from build123d import *

# Parameters (mm, degrees)
BOSS_EXTRUDE3_DEPTH = 13
FILLET1_R           = 1
FILLET2_R           = 5
SKETCH2_R           = 2.4
CUT_EXTRUDE1_DEPTH  = 7.5
FILLET3_R           = 2.5


with BuildPart() as part:
    # Sketch1 → Boss-Extrude3 (new body)
    with BuildSketch(Plane.XY):
        Polygon((-12.5, 10.5), (-4.45, 10.5), (4.45, 10.5), (12.5, 10.5), (12.5, 24.5), (-12.5, 33.5), align=None)
        Polygon((-4.45, 7.3), (-10.25, 7.3), (-4, 0), (4, 0), (10.25, 7.3), (4.45, 7.3), (4.45, 10.5), (-4.45, 10.5), align=None)
    extrude(amount=BOSS_EXTRUDE3_DEPTH)

    # Fillet1
    fillet1_edges = [part.edges().sort_by_distance(p)[0] for p in [
        (10.25, 7.3, 6.5),
        (-10.25, 7.3, 6.5),
    ]]
    fillet(fillet1_edges, radius=FILLET1_R)

    # Fillet2
    fillet2_edges = [part.edges().sort_by_distance(p)[0] for p in [
        (4, 0, 6.5),
        (-4, 0, 6.5),
    ]]
    fillet(fillet2_edges, radius=FILLET2_R)

    # Sketch2 → Cut-Extrude1 (cut)
    with BuildSketch(Plane(origin=(9.242209632, 25.672804533, 0), x_dir=(0.9408874118687268, -0.33871946827274163, 0), z_dir=(0.33871946827274163, 0.9408874118687268, 0))):
        with Locations(Location((-17.537534324, -6.5, 0), (0, 0, 180))):
            Circle(SKETCH2_R)
        with Locations(Location((-2.537534324, -6.5, 0), (0, 0, 180))):
            Circle(SKETCH2_R)
    extrude(amount=-CUT_EXTRUDE1_DEPTH, mode=Mode.SUBTRACT)

    # Fillet3
    fillet3_edges = [part.edges().sort_by_distance(p)[0] for p in [
        (-12.5, 22, 13),
        (-12.5, 22, 0),
        (12.5, 17.5, 0),
        (12.5, 17.5, 13),
    ]]
    fillet(fillet3_edges, radius=FILLET3_R)


solid = part.part
Can you work these out from the model? Positions are in its coordinate system, mm. A direction names the side the tool comes from. Coordinates: 2 decimals unless noted, no trailing zeros. Write each loop counter-clockwise with the first axis right and the second up, starting at its lowest first coordinate (ties: lowest second). Pieces come first, ordered by that corner, then holes. Notation, with made-up numbers: (56.25, -14) - (103.25, -14) arc R29 ccw to (103.25, 24) - close; hole circle Ø11 at (-16.5, 87.25). An arc over 180 degrees is marked (long way). Return JSON: item names as keys, results as strings. Group by question number.
Item 1: I'm going to push flat-ended pins straight in: pin 1 Ø3.5 at (y, z) = (9.5, 7) entering from -X; pin 2 Ø6 at (x, z) = (9, 9.5) entering from +Y; pin 3 Ø4 at (x, z) = (-7, 8) entering from +Y; pin 4 Ø4 at (x, z) = (7.5, 3) entering from -Y. Where does each tip first touch, or does it pass through?
Item 2: Which directions (+Z, -Z, +X, -X, +Y, -Y) give clear straight access to the entire face, cutting with the end or side of a thin tool? Please do faces 1 (the face through (-6, 7.3, 6)), 2 (the face through (6, 7.3, 6)), 3 (the face through (-7.19, 3.726, 6.409)), 4 (the face through (-9.767, 24.545, 6.534)), 5 (the face through (7.14, 3.67, 6.41)).
Item 3: If we section it at C-C (z = 1): Write out the boundary of the cut face in (x, y), then the cut area to 3 significant figures.
Item 4: We'd pull the mould along X, two halves only. Please class faces 6 (the face through (4.45, 9, 6)), 7 (the face through (-6.255, 27.322, 6.606)), 8 (the face through (-12, 22, 12)): pulls with the +X half, pulls with the -X half, needs draft (parallel to the pull), parting line crosses it, or undercut.
Item 5: If we section it at B-B (z = 3): Write out the boundary of the cut face in (x, y).
Item 6: If we section it at A-A (y = 16): Write out the boundary of the cut face in (x, z), then the cut area to 3 significant figures.
Item 7: If we section it at D-D (z = 8.5): Write out the boundary of the cut face in (x, y), then the cut area to 3 significant figures.
Item 8: Please list where these lines run through material, in increasing order: probe 1 along Y at (x, z) = (8.5, 10); probe 2 along Y at (x, z) = (7, 2.5); probe 3 along Z at (x, y) = (-7, 27.5).
Return value:
{
 "1": {"pin 1": "stops at x = -12.5", "pin 2": "stops at y = 26.84", "pin 3": "stops at y = 32.24", "pin 4": "stops at y = 1.75"},
 "2": {"face 1": "+Z, -Z, -X", "face 2": "+Z, -Z, +X", "face 3": "+Z, -Z, -X, -Y", "face 4": "none", "face 5": "+Z, -Z, +X, -Y"},
 "3": {"outline": "(-12, 10.5) - (-4.45, 10.5) - (-4.45, 7.3) - (-8.08, 7.3) arc R1 ccw to (-8.84, 5.65) - (-5.5, 1.75) arc R5 ccw to (-1.7, 0) - (1.7, 0) arc R5 ccw to (5.5, 1.75) - (8.84, 5.65) arc R1 ccw to (8.08, 7.3) - (4.45, 7.3) - (4.45, 10.5) - (12, 10.5) - (12, 24.68) - (-12, 33.32) - close", "area": "573 mm^2"},
 "4": {"face 6": "pulls with the +X half", "face 7": "undercut", "face 8": "pulls with the -X half"},
 "5": {"outline": "(-12.5, 10.5) - (-4.45, 10.5) - (-4.45, 7.3) - (-8.08, 7.3) arc R1 ccw to (-8.84, 5.65) - (-5.5, 1.75) arc R5 ccw to (-1.7, 0) - (1.7, 0) arc R5 ccw to (5.5, 1.75) - (8.84, 5.65) arc R1 ccw to (8.08, 7.3) - (4.45, 7.3) - (4.45, 10.5) - (12.5, 10.5) - (12.5, 24.5) - (-12.5, 33.5) - close"},
 "6": {"outline": "(-12.5, 2.5) arc R2.5 ccw to (-10, 0) - (10, 0) arc R2.5 ccw to (12.5, 2.5) - (12.5, 10.5) arc R2.5 ccw to (10, 13) - (-10, 13) arc R2.5 ccw to (-12.5, 10.5) - close", "area": "320 mm^2"},
 "7": {"outline": "(-12.5, 10.5) - (-4.45, 10.5) - (-4.45, 7.3) - (-8.08, 7.3) arc R1 ccw to (-8.84, 5.65) - (-5.5, 1.75) arc R5 ccw to (-1.7, 0) - (1.7, 0) arc R5 ccw to (5.5, 1.75) - (8.84, 5.65) arc R1 ccw to (8.08, 7.3) - (4.45, 7.3) - (4.45, 10.5) - (12.5, 10.5) - (12.5, 24.5) - (8.1, 26.08) - (5.56, 19.03) - (3.07, 19.93) - (5.61, 26.98) - (-6.01, 31.16) - (-8.55, 24.11) - (-11.05, 25.01) - (-8.51, 32.06) - (-12.5, 33.5) - close", "area": "552 mm^2"},
 "8": {"probe 1": "y = 5.26 to 7.21, 10.5 to 25.94", "probe 2": "y = 3.5 to 7.3, 10.5 to 26.48", "probe 3": "z = 0 to 4.74, 8.26 to 13"}
}
